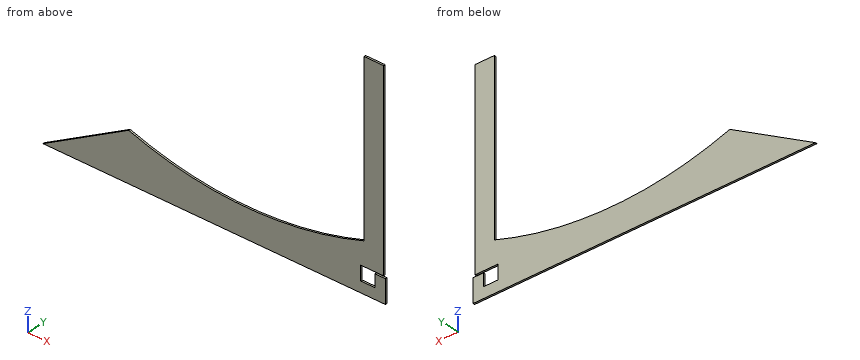
```python
from build123d import *

# Parameters (mm, degrees)
F1_DEPTH = 6.35
F2_W     = 6.35
F2_H     = 673.1
F3_DEPTH = 25.4


with BuildPart() as f1:
    # F0 (on Front) → F1 (new body)
    with BuildSketch(Plane.XZ):
        Polygon((304.8, 171.45), (0, 0), (1219.2, 0), (1219.2, 762), (1143, 762), (1143, 171.45), (1143, 101.6), (723.9, 101.6), (306.02731713, 101.6), (303.9947166863, 99.612464416), (268.4785905511, 135.9338738649), align=None)
        with BuildLine():
            ThreePointArc((723.9, 101.6), (511.4595186293, 119.182111776), (304.8, 171.45))
            Line((304.8, 171.45), (340.3161261351, 135.1285905511))
            Line((340.3161261351, 135.1285905511), (306.02731713, 101.6))
            Line((306.02731713, 101.6), (723.9, 101.6))
        make_face()
        with BuildLine():
            ThreePointArc((1143, 171.45), (936.3404813707, 119.182111776), (723.9, 101.6))
            Line((723.9, 101.6), (1143, 101.6))
            Line((1143, 101.6), (1143, 171.45))
        make_face()
        Polygon((304.8, 101.6), (304.8, 171.45), (268.4785905511, 135.9338738649), (303.9947166863, 99.612464416), (306.02731713, 101.6), align=None)
        Polygon((340.3161261351, 135.1285905511), (304.8, 171.45), (304.8, 101.6), (306.02731713, 101.6), align=None)
    extrude(amount=F1_DEPTH)

    # F2 (on face) → F3 (cut)
    with BuildSketch(Plane.XZ.offset(6.35)):
        Polygon((1130.3, 88.9), (1130.3, 38.1), (1181.1, 38.1), (1181.1, 82.55), (1181.1, 88.9), align=None)
        with Locations((1216.025, 425.45)):
            Rectangle(F2_W, F2_H)
        Polygon((1181.1, 88.9), (1181.1, 82.55), (1219.2, 82.55), (1219.2, 88.9), (1212.85, 88.9), align=None)
    extrude(amount=-F3_DEPTH, mode=Mode.SUBTRACT)


solid = f1.part
```
For this review, take the finished solid that the model builds, in its own axes (mm). Give positions to 0.01 mm unless a question says otherwise; leave off trailing zeros. Write each loop counter-clockwise with the first axis right and the second up, starting at its lowest first coordinate (ties: lowest second). Pieces come first, ordered by that corner, then holes. Notation, with made-up numbers: M 85,77.25 L 111,77.25 A26 cw 111,95.25 Z; hole C 32,14 d4. An arc over 180 degrees is marked long. Answer as CSV lines item,"result".
1. Consider section A-A, the plane z = 126. Write out the cut boundary in (x, y).
Findings:
outline,"M 224,-6.35 L 473.97,-6.35 L 473.97,0 L 224,0 Z; M 973.83,-6.35 L 1212.85,-6.35 L 1212.85,0 L 973.83,0 Z"
2. Consider section B-B, the plane y = -4. Write out the cut boundary in (x, z) (3 decimals), then the cut area to 3 significant figures.
Findings:
outline,"M 0,0 L 1219.2,0 L 1219.2,82.55 L 1181.1,82.55 L 1181.1,38.1 L 1130.3,38.1 L 1130.3,88.9 L 1212.85,88.9 L 1212.85,762 L 1143,762 L 1143,171.45 A1292.225 cw 304.8,171.45 Z"
area,"182,000 mm2"
3. Consider section D-D, the plane x = 578. Write out the cut boundary in (y, z), then the cut area to 3 significant figures.
Findings:
outline,"M -6.35,0 L 0,0 L 0,109.86 L -6.35,109.86 Z"
area,"698 mm2"
4. Wall thickness on line 1 (Z direction, x = 1163, y = -2.5); line 2 (X direction, y = -0.5, z = 192.5): over which ranges is each line inside the solid? List them lowest first.
Findings:
line 1,"z = 0 to 38.1, 88.9 to 762"
line 2,"x = 1143 to 1212.85"
5. Consider section C-C, the plane z = 711.5. Write out the cut boundary in (x, y).
Findings:
outline,"M 1143,-6.35 L 1212.85,-6.35 L 1212.85,0 L 1143,0 Z"
6. For pin 1 (3 mm diameter, centred on y = -5.5, z = 482.5, fed in from +X); pin 2 (2 mm diameter, centred on x = 210.5, y = -2, fed in from +Z); pin 3 (3 mm diameter, centred on y = -1.5, z = 423, fed in from -X), all flat-tipped, find the tip position at first contact; note any pin that passes through.
Findings:
pin 1,"stops at x = 1212.85"
pin 2,"stops at z = 118.97"
pin 3,"stops at x = 1143"
